from build123d import *

# Parameters (mm, degrees)
SKETCH1_R               = 18.2
BOSS_EXTRUDE1_DEPTH     = 5.6
CUT_EXTRUDE1_DEPTH      = 4
SKETCH3_R               = 3.5
CUT_EXTRUDE2_DEPTH      = 0.75
CUT_EXTRUDE3_REACH      = 44.811
CUT_EXTRUDE3_END_RADIUS = 18.2
CUT_EXTRUDE3_START      = 16.47
SKETCH5_W               = 3
SKETCH5_H               = 6.8


with BuildPart() as part:
    # Sketch1 → Boss-Extrude1 (new body)
    with BuildSketch(Plane.XY):
        Circle(SKETCH1_R)
    extrude(amount=BOSS_EXTRUDE1_DEPTH)

    # Sketch2 → Cut-Extrude1 (cut)
    with BuildSketch(Plane(origin=(0, 0, 0), x_dir=(-1, 0, 0), z_dir=(0, 0, -1))):
        with BuildLine():
            ThreePointArc((12.962542311, -11.756806404), (13.503430209, -11.131368855), (14.014170433, -10.481079481))
            ThreePointArc((14.014170433, -10.481079481), (13.929523254, -10.546491611), (13.823271504, -10.558919696))
            ThreePointArc((13.823271504, -10.558919696), (13.129289386, -10.822950961), (13.00252715, -11.554562213))
            ThreePointArc((13.00252715, -11.554562213), (13.010601193, -11.661233209), (12.962542311, -11.756806404))
        make_face()
        with BuildLine():
            ThreePointArc((-12.406576366, -12.133139552), (-10.177222153, -12.345957703), (-9.542933233, -14.493744783))
            ThreePointArc((-9.542933233, -14.493744783), (-9.540416363, -14.622080688), (-9.460407641, -14.722455205))
            ThreePointArc((-9.460407641, -14.722455205), (-11.131368855, -13.503430209), (-12.646831358, -12.095770194))
            ThreePointArc((-12.646831358, -12.095770194), (-12.53303462, -12.155156569), (-12.406576366, -12.133139552))
        make_face()
        with BuildLine():
            ThreePointArc((12.406576366, 12.133139552), (12.53303462, 12.155156569), (12.646831358, 12.095770194))
            ThreePointArc((12.646831358, 12.095770194), (11.131368855, 13.503430209), (9.460407641, 14.722455205))
            ThreePointArc((9.460407641, 14.722455205), (9.540416363, 14.622080688), (9.542933233, 14.493744783))
            ThreePointArc((9.542933233, 14.493744783), (10.177222153, 12.345957703), (12.406576366, 12.133139552))
        make_face()
    extrude(amount=-CUT_EXTRUDE1_DEPTH, mode=Mode.SUBTRACT)

    # Sketch3 → Cut-Extrude2 (cut)
    with BuildSketch(Plane.XY.offset(5.6)):
        Circle(SKETCH3_R)
    extrude(amount=-CUT_EXTRUDE2_DEPTH, mode=Mode.SUBTRACT)

    # Cut-Extrude3: up to this cylinder (the profile starts inside it)
    cut_extrude3_end = Plane(origin=(0, 0, 2.8), z_dir=(0, 0, -1)) * Cylinder(CUT_EXTRUDE3_END_RADIUS, 127.022, mode=Mode.PRIVATE)
    # Sketch5 → Cut-Extrude3 (cut, up to the surface)
    with BuildSketch(Plane(origin=(0, 0, 0), x_dir=(0, 0, -1), z_dir=(-0.25881904510252135, 0.9659258262890681, 0)).offset(CUT_EXTRUDE3_START), mode=Mode.PRIVATE) as cut_extrude3_sk1:
        with Locations((-2.8, 0)):
            Rectangle(SKETCH5_W, SKETCH5_H)
    cut_extrude3_tool1 = extrude(cut_extrude3_sk1.sketch, amount=CUT_EXTRUDE3_REACH, mode=Mode.PRIVATE) & cut_extrude3_end
    add(cut_extrude3_tool1.solids().sort_by_distance((-4.26275, 15.908798, 2.8))[0], mode=Mode.SUBTRACT)


solid = part.part
Build history of the part. All positions in model axes, mm. A direction names the side the tool comes from. Round coordinates to 2 decimals unless told otherwise and drop trailing zeros. Write each loop counter-clockwise with the first axis right and the second up, starting at its lowest first coordinate (ties: lowest second). Pieces come first, ordered by that corner, then holes. Notation, with made-up numbers: (25, 26) -> (35, 26) arc R28 cw to (35, 55) -> close; hole circle Ø1 at (-9.5, 63). An arc over 180 degrees is marked (long way). Write item = value, one per line.
(1) Two-plate mould, pull along Y, no slides. Class faces 6 (the face through (0, 0, 0)), 7 (the face through (-7.727, 15.7, 2.821)), 8 (the face through (11.11, -13.52, 1.97)), 9 (the face through (-10.15, 12.37, 1.97)): pulls with the +Y half, pulls with the -Y half, needs draft (parallel to the pull), parting line crosses it, or undercut.
Answer:
face_6 = needs draft
face_7 = pulls with the +Y half
face_8 = undercut
face_9 = undercut
(2) Tool access for faces 1 (the face through (10.2, -12.33, 1.97)), 2 (the face through (-1.16, 17.46, 2.82)), 3 (the face through (0, -4, 5.6)), 4 (the face through (3.233, -1.341, 5.23)), 5 (the face through (-3.945, -17.767, 2.761)): list every direction of +Z, -Z, +X, -X, +Y, -Y with a clear straight run to the whole face (end or side of a thin tool).
Answer:
face_1 = -Z
face_2 = -X
face_3 = +Z, +X, -X, +Y, -Y
face_4 = +Z
face_5 = +Z, -Z
(3) Band-saw the part on D-D (x = 15). Give the cut face in (y, z).
Answer:
outline = (-10.31, 0) -> (10.31, 0) -> (10.31, 5.6) -> (-10.31, 5.6) -> close
(4) Probe L1, parallel to Y at x = 0, z = 5.3; L2, parallel to Y at x = -12, z = 1.4; L3, parallel to X at y = 3, z = 2.15. List the from-to ranges inside material, lowest first.
Answer:
L1 = -18.2 to -3.5, 3.5 to 18.2
L2 = -13.68 to 11.97, 12.74 to 13.68
L3 = -17.95 to 17.95
(5) Flat gauge pins, fed straight in: pin 1 (1 mm diameter, centred on y = 2, z = 3.5, fed in from -X); pin 2 (4 mm diameter, centred on x = 0, y = 0, fed in from +Z); pin 3 (2 mm diameter, centred on x = 2.5, z = 3, fed in from -Y). Where does each tip first touch, or does it go through?
Answer:
pin_1 = -18.14
pin_2 = 4.85
pin_3 = -18.14
(6) Band-saw the part on C-C (x = 4). Give the cut face in (y, z) (3 decimals), then the cut area to 3 significant figures.
Answer:
outline = (-17.755, 0) -> (17.755, 0) -> (17.755, 5.6) -> (-17.755, 5.6) -> close
area = 199 mm2
(7) Band-saw the part on A-A (x = 0). Give the cut face in (y, z), then the cut area to 3 significant figures.
Answer:
outline = (-18.2, 0) -> (18.2, 0) -> (18.2, 5.6) -> (3.5, 5.6) -> (3.5, 4.85) -> (-3.5, 4.85) -> (-3.5, 5.6) -> (-18.2, 5.6) -> close
area = 199 mm2
